Solid Edge part; units mm, degrees
sketch "Sketch1" plane through (0, 0, 0) normal (0, 0, 1) x (1, 0, 0)
  circle A0 centre (0, 0) radius 2.725
extrude "Protrusion1" add sketch "Sketch1" against normal blind 3
sketch "Sketch2" plane through (0, 0, 0) normal (0, 0, 1) x (1, 0, 0)
  line L0 (-0.7, -1.2124) -> (-1.05, -0.6062)
  line L1 (-1.4, 0) -> (-1.05, -0.6062)
  line L2 (-1.4, 0) -> (-1.05, 0.6062)
  line L3 (-0.7, 1.2124) -> (-1.05, 0.6062)
  line L4 (-0.7, 1.2124) -> (0, 1.2124)
  line L5 (0.7, 1.2124) -> (0, 1.2124)
  line L6 (0.7, 1.2124) -> (1.05, 0.6062)
  line L7 (1.4, 0) -> (1.05, 0.6062)
  line L8 (1.4, 0) -> (1.05, -0.6062)
  line L9 (0.7, -1.2124) -> (1.05, -0.6062)
  line L10 (0.7, -1.2124) -> (0, -1.2124)
  line L11 (-0.7, -1.2124) -> (0, -1.2124)
extrude "ExtrudedCutout_1" cut sketch "Sketch2" against normal blind 1.45
sketch "Sketch3" plane through (0, 0, -3) normal (0, 0, -1) x (1, 0, 0)
  circle A0 centre (0, 0) radius 1.5
extrude "ExtrudedProtrusion_2" add sketch "Sketch3" along normal blind 25
cosmetic_thread "Thread_2" thread depth 17
Geometry: final body of the model. Coordinates: model frame, mm. A direction names the side the tool comes from. Give positions to 0.01 mm unless a question says otherwise; leave off trailing zeros. Write each loop counter-clockwise with the first axis right and the second up, starting at its lowest first coordinate (ties: lowest second). Pieces come first, ordered by that corner, then holes.
(1) Cut plane B-B, the plane z = -23.25. Return loops of the section in (x, y), then the cut area to 3 significant figures.
(2) Mould query, pull axis X, two halves, no side actions, for faces 4 (the cylindrical face through (-1.5, 0.07, -15.32)), 5 (the flat face through (1.05, -0.61, -0.71)), 6 (the flat face through (0, 0, -1.45)), 7 (the flat face through (1, -1, 0)). Classes: released by +X, released by -X, zero draft, split by the parting line, or undercut.
(3) Access query for faces 1 (the flat face through (0, 0, -28)), 2 (the flat face through (0, -1.212, -1)), 3 (the flat face through (1.2, -1.2, -3)). Directions: +Z, -Z, +X, -X, +Y, -Y. A direction counts if a zero-diameter tool reaches every point of the face in a straight line with its end or side. Return the directions, or none.
(4) First-contact query: P1, Ø2.5, axis at x = -0.5, y = -0.5, coming from the +Z side; P2, Ø3, axis at y = -0.5, z = -8.5, coming from the +X side; P3, Ø1.5, axis at y = 0, z = -7, coming from the -X side. Flat tips, straight axial feed; report the tip coordinate or a pass-through.
(5) Cut plane D-D, the plane x = 1.05. Return loops of the section in (y, z), then the cut area to 3 significant figures.
(6) Cut plane C-C, the plane y = -1.85. Return loops of the section in (x, z), then the cut area to 3 significant figures.
(7) Cut plane A-A, the plane x = 0. Return loops of the section in (y, z) (3 decimals), then the cut area to 3 significant figures.
(8) Ray query, line 1 (Z direction, x = -1.95, y = -0.15); line 2 (Z direction, x = -0.75, y = -0.9); line 3 (X direction, y = -0.05, z = -17). Return the intervals inside material, ascending.
Values follow:
1. outline: circle Ø3 at (0, 0)
1. area: 7.07 mm2
2. face 4: split by the parting line
2. face 5: undercut
2. face 6: undercut
2. face 7: zero draft
3. face 1: -Z, +X, -X, +Y, -Y
3. face 2: +Z
3. face 3: -Z
4. P1: stops at z = 0
4. P2: stops at x = 1.5
4. P3: stops at x = -1.5
5. outline: (-2.51, -3) - (-1.07, -3) - (-1.07, -28) - (1.07, -28) - (1.07, -3) - (2.51, -3) - (2.51, 0) - (0.61, 0) - (0.61, -1.45) - (-0.61, -1.45) - (-0.61, 0) - (-2.51, 0) - close
5. area: 66.9 mm2
6. outline: (-2, -3) - (2, -3) - (2, 0) - (-2, 0) - close
6. area: 12.0 mm2
7. outline: (-2.725, -3) - (-1.5, -3) - (-1.5, -28) - (1.5, -28) - (1.5, -3) - (2.725, -3) - (2.725, 0) - (1.212, 0) - (1.212, -1.45) - (-1.212, -1.45) - (-1.212, 0) - (-2.725, 0) - close
7. area: 87.8 mm2
8. line 1: z = -3 to 0
8. line 2: z = -28 to -1.45
8. line 3: x = -1.5 to 1.5
